from build123d import *

# Parameters (mm, degrees)
SKETCH1_W           = 28
SKETCH1_H           = 20
BOSS_EXTRUDE1_DEPTH = 3
SKETCH2_W           = 3
SKETCH2_H           = 20
BOSS_EXTRUDE2_DEPTH = 25
SKETCH3_W           = 25
SKETCH3_H           = 3
BOSS_EXTRUDE3_DEPTH = 25
CUT_EXTRUDE1_DEPTH  = 25
CUT_EXTRUDE2_DEPTH  = 25
CUT_EXTRUDE3_DEPTH  = 25
CUT_EXTRUDE4_DEPTH  = 25


with BuildPart() as part:
    # Sketch1 → Boss-Extrude1 (new body)
    with BuildSketch(Plane(origin=(0, 0, 0), x_dir=(1, 0, 0), z_dir=(0, 1, 0))):
        with Locations((0.825174825, 2.237762238)):
            Rectangle(SKETCH1_W, SKETCH1_H)
    extrude(amount=BOSS_EXTRUDE1_DEPTH)

    # Sketch2 → Boss-Extrude2 (add)
    with BuildSketch(Plane(origin=(0, 3, 0), x_dir=(1, 0, 0), z_dir=(0, 1, 0))):
        with Locations((-11.674825175, 2.237762238)):
            Rectangle(SKETCH2_W, SKETCH2_H)
    extrude(amount=BOSS_EXTRUDE2_DEPTH)

    # Sketch3 → Boss-Extrude3 (add)
    with BuildSketch(Plane(origin=(0, 3, 0), x_dir=(1, 0, 0), z_dir=(0, 1, 0))):
        with Locations((2.325174825, -6.262237762)):
            Rectangle(SKETCH3_W, SKETCH3_H)
        with Locations((2.325174825, 10.737762238)):
            Rectangle(SKETCH3_W, SKETCH3_H)
    extrude(amount=BOSS_EXTRUDE3_DEPTH)

    # Sketch4 → Cut-Extrude1 (cut)
    with BuildSketch(Plane.XY.offset(-9.237762238)):
        with BuildLine():
            add(Edge.make_bspline(
                [(14.816368242, 3.008806583), (6.487903216, 11.337271609), (-1.840561809, 19.665736635), (-10.169026835, 27.99420166), (-10.16964342, 27.994818245), (-10.170781245, 27.99595607), (-10.170656704, 27.998996051), (-10.170343396, 28)],
                knots=[0, 0, 0, 0, 0.344046384, 0.344046384, 0.344046384, 0.344071855, 0.344093387, 0.344093387, 0.344093387, 0.344093387], degree=3))
            add(Edge.make_bspline(
                [(14.825174825, 3.004378162), (14.823896916, 3.004464678), (14.819965163, 3.005209662), (14.817823619, 3.007351206), (14.816368242, 3.008806583)],
                knots=[0.999911533, 0.999911533, 0.999911533, 0.999911533, 0.999939879, 1, 1, 1, 1], degree=3))
            Line((14.825174825, 3.004378162), (14.825174825, 28))
            Line((14.825174825, 28), (-10.170343396, 28))
        make_face()
    extrude(amount=-CUT_EXTRUDE1_DEPTH, mode=Mode.SUBTRACT)

    # Sketch5 → Cut-Extrude2 (cut)
    with BuildSketch(Plane(origin=(0, 0, 4.762237762), x_dir=(-1, 0, 0), z_dir=(0, 0, -1))):
        with BuildLine():
            add(Edge.make_bspline(
                [(-35.067252589, 33.961212886), (-29.391038068, 36.178470487), (-23.714823548, 38.395728089), (-18.038609027, 40.612985691), (-17.963791349, 40.642211165), (-17.814155994, 40.700662115), (-17.559065615, 40.718177611), (-17.399544187, 40.699199542), (-17.319783474, 40.689710508), (-10.209359532, 39.843792085), (-3.09893559, 38.997873662), (4.011488351, 38.151955239), (4.046454663, 38.14779534), (4.116387287, 38.139475541), (4.223224946, 38.0698289), (4.25905817, 38.009200763), (4.276974782, 37.978886695), (6.22420547, 34.684263552), (8.171436157, 31.389640408), (10.118666845, 28.095017265), (10.128528722, 28.078331431), (10.148252475, 28.044959763), (10.137896266, 27.963071091), (10.11048555, 27.935660375), (10.096780192, 27.921955017), (1.809823102, 19.634997927), (-6.477133988, 11.348040838), (-14.764091077, 3.061083748), (-14.773689462, 3.051485363), (-14.792886232, 3.032288593), (-14.857463418, 3.032288593), (-14.876660188, 3.051485363), (-14.886258573, 3.061083748), (-16.63085756, 4.805682735), (-18.375456547, 6.550281721), (-20.120055533, 8.294880708), (-20.229166807, 8.403991982), (-20.447389354, 8.622214529), (-20.734044746, 8.995724629), (-20.888397332, 9.262965044), (-20.965573625, 9.396585251), (-25.677007414, 17.553789146), (-30.388441203, 25.71099304), (-35.099874992, 33.868196935), (-35.105352774, 33.877680966), (-35.116308338, 33.896649028), (-35.097857424, 33.949257946), (-35.077454201, 33.957227906), (-35.067252589, 33.961212886)],
                knots=[0, 0, 0, 0, 0.146383908, 0.146383908, 0.146383908, 0.148313382, 0.150242855, 0.152172328, 0.152172328, 0.152172328, 0.324178973, 0.324178973, 0.324178973, 0.325024835, 0.325870697, 0.326716559, 0.326716559, 0.326716559, 0.418647366, 0.418647366, 0.418647366, 0.419112956, 0.419578546, 0.420044135, 0.420044135, 0.420044135, 0.701563293, 0.701563293, 0.701563293, 0.701889363, 0.702215434, 0.702541504, 0.702541504, 0.702541504, 0.761807895, 0.761807895, 0.761807895, 0.765514552, 0.76922121, 0.772927868, 0.772927868, 0.772927868, 0.999210732, 0.999210732, 0.999210732, 0.999473821, 0.999736911, 1, 1, 1, 1], degree=3))
        make_face()
    extrude(amount=-CUT_EXTRUDE2_DEPTH, mode=Mode.SUBTRACT)

    # Sketch6 → Cut-Extrude3 (cut)
    with BuildSketch(Plane(origin=(-10.174825175, 0, 0), x_dir=(0, 0, -1), z_dir=(1, 0, 0))):
        with BuildLine():
            Line((-0.762237762, 11), (-0.762237762, 20))
            ThreePointArc((-0.762237762, 20), (2.237762238, 23), (5.237762238, 20))
            Line((5.237762238, 20), (5.237762238, 11))
            ThreePointArc((5.237762238, 11), (2.237762238, 8), (-0.762237762, 11))
        make_face()
    extrude(amount=-CUT_EXTRUDE3_DEPTH, mode=Mode.SUBTRACT)

    # Sketch7 → Cut-Extrude4 (cut)
    with BuildSketch(Plane(origin=(0, 3, 0), x_dir=(1, 0, 0), z_dir=(0, 1, 0))):
        with BuildLine():
            Line((6.643802614, -0.720378412), (-2.16057373, -0.762203911))
            ThreePointArc((-2.16057373, -0.762203911), (-5.174791324, 2.223510793), (-2.189076619, 5.237728387))
            Line((-2.189076619, 5.237728387), (6.615299725, 5.279553886))
            ThreePointArc((6.615299725, 5.279553886), (9.629517318, 2.293839181), (6.643802614, -0.720378412))
        make_face()
    extrude(amount=-CUT_EXTRUDE4_DEPTH, mode=Mode.SUBTRACT)


solid = part.part
Can you work these out from the model? Positions are in its coordinate system, mm. A direction names the side the tool comes from. Coordinates: 2 decimals unless noted, no trailing zeros. Loops run counter-clockwise (first coordinate to the right, second up) from the corner with the lowest first, then second, coordinate; pieces in that order, holes last. Notation, with made-up numbers: M -20.75,80 L 32.25,80 A13 cw 32.25,87 Z; hole C -15.75,-9 d1. An arc over 180 degrees is marked long. Return JSON: item names as keys, results as strings. Group by question number.
Item 1: Thinking about a two-plate mould opening in X: for faces 1 (the flat face through (-1, 13, -9.238)), 2 (the cylindrical face through (9.63, 1.52, -2.36)), 3 (the flat face through (-13.175, 14, 2)), which applies, released by +X, released by -X, zero draft, split by the parting line, or undercut?
Item 2: If I drill on L1, parallel to Z at x = -7.25, y = 19.25; L2, parallel to Z at x = 5, y = 2.75; L3, parallel to Y at x = 4.75, z = 3.75, over which ranges is the centre line in solid material (lowest first)? Write a range as from..to.
Item 3: On a 3-axis mill with a long thin cutter (end or side, diameter ignored), from which of +Z, -Z, +X, -X, +Y, -Y can I reach the whole of each face in a straight line? I mean faces 4 (the flat face through (-12, 16, -5.238)), 5 (the cylindrical face through (-5.174, 1.521, -2.158)), 6 (the flat face through (-10.175, 15, 1)). Say none if no direction works.
Item 4: Imagine slicing it at B-B (z = -7.5). Please give me the cut outline in (x, y), and give its area (3 significant figures).
Item 5: I'm going to push flat-ended pins straight in: pin 1 Ø5 at (x, y) = (5.5, 16) entering from -Z; pin 2 Ø4 at (y, z) = (22.5, 4) entering from +X; pin 3 Ø6 at (x, z) = (9.5, -2.5) entering from +Y; pin 4 Ø3 at (y, z) = (22, 5.5) entering from +X. Where does each tip first touch, or does it pass through?
Item 6: Imagine slicing it at A-A (z = -2.5). Please give me the cut outline in (x, y), and give its area (3 significant figures).
Verdict:
{
 "1": {"face 1": "zero draft", "face 2": "undercut", "face 3": "released by -X"},
 "2": {"L1": "z = -12.24..-9.24, 4.76..7.76", "L2": "z = -12.24..-5.27, 0.73..7.76", "L3": "y = 0..3"},
 "3": {"face 4": "+X, -X", "face 5": "+Y, -Y", "face 6": "+X, +Y"},
 "4": {"outline": "M -13.17,0 L 14.83,0 L 14.83,3 L -10.17,3 L -10.17,28 L -13.17,28 Z", "area": "159 mm^2"},
 "5": {"pin 1": "passes through", "pin 2": "stops at x = -2.83", "pin 3": "stops at y = 3", "pin 4": "stops at x = -2.67"},
 "6": {"outline": "M -13.17,0 L -5.16,0 L -5.16,3 L -10.17,3 L -10.17,8.01 L -13.17,8.01 Z; M -13.17,22.99 L -10.17,22.99 L -10.17,28 L -13.17,28 Z; M 9.62,0 L 14.83,0 L 14.83,3 L 9.62,3 Z", "area": "69.7 mm^2"}
}
